from build123d import *

# Parameters (mm, degrees)
SKETCH_1_R      = 2.5
SKETCH_1_R_2    = 2
EXTRUDE_1_DEPTH = 5
SKETCH_2_R      = 2.75
SKETCH_2_R_2    = 2.25
EXTRUDE_2_DEPTH = 6
FILLET_1_R      = 0.1


with BuildPart() as part:
    # Эскиз1 → Вытянуть1 (new body)
    with BuildSketch(Plane.XY):
        Circle(SKETCH_1_R)
        Circle(SKETCH_1_R_2, mode=Mode.SUBTRACT)
    extrude(amount=EXTRUDE_1_DEPTH)

    # Эскиз2 → Вытянуть2 (add)
    with BuildSketch(Plane.XY.offset(5)):
        Circle(SKETCH_2_R)
        Circle(SKETCH_2_R_2, mode=Mode.SUBTRACT)
    extrude(amount=EXTRUDE_2_DEPTH)

    # Скругление1
    fillet_1_edges = [part.edges().sort_by_distance(p)[0] for p in [
        (-2.5, 0, 0),
        (-2.5, 0, 5),
        (-2.75, 0, 5),
    ]]
    fillet(fillet_1_edges, radius=FILLET_1_R)


solid = part.part
Design review of the part built by this model. Coordinates are the model's own, in mm. A direction names the side the tool comes from. Coordinates: 2 decimals unless noted, no trailing zeros. Order: outer loops, then holes, each group sorted by start corner. A loop starts at its lowest first (then second) coordinate and runs counter-clockwise, first axis right, second up.
Item 1: For line 1 (Y direction, x = 0, z = 7.6); line 2 (Y direction, x = 0, z = 1.6); line 3 (X direction, y = -1.5, z = 1.25), list the stretches that pass through material, from the lowest coordinate up.
Item 2: The part is to be moulded in two halves that separate along X. For faces 1 (the cylindrical face through (-0.29, 2.23, 7.96)), 2 (the flat face through (-1, 2, 0)), 3 (the cylindrical face through (-0.596, -2.685, 8.009)), say which applies: pulls with the +X half, pulls with the -X half, needs draft (parallel to the pull), parting line crosses it, or undercut.
Item 3: Take a section at D-D, the plane z = 3.75. Write out the cut boundary in (x, y), then the cut area to 3 significant figures.
Item 4: Take a section at C-C, the plane z = 9.75. Write out the cut boundary in (x, y).
Item 5: For faces 4 (the cylindrical face through (0, -2, 2)), 5 (the cylindrical face through (-0.54, -2.44, 2.47)), list the 3-axis set-ups (+Z, -Z, +X, -X, +Y, -Y) from which the entire face can be reached by the end or side of a thin tool; tool diameter is ignored.
Item 6: Take a section at A-A, the plane y = 0. Write out the cut boundary in (x, z), then the cut area to 3 significant figures.
Item 7: For pin 1 Ø2 at (y, z) = (-0.5, 5) entering from -X; pin 2 Ø2 at (x, z) = (-2, 8.5) entering from -Y; pin 3 Ø2 at (x, y) = (-1, 0.5) entering from +Z; pin 4 Ø1.6 at (x, y) = (0.5, -1) entering from -Z, all flat-tipped, find the tip position at first contact; note any pin that passes through.
The answers:
1. line 1: y = -2.75 to -2.25, 2.25 to 2.75
1. line 2: y = -2.5 to -2, 2 to 2.5
1. line 3: x = -2 to -1.32, 1.32 to 2
2. face 1: undercut
2. face 2: needs draft
2. face 3: parting line crosses it
3. outline: circle Ø5 at (0, 0); hole circle Ø4 at (0, 0)
3. area: 7.07 mm2
4. outline: circle Ø5.5 at (0, 0); hole circle Ø4.5 at (0, 0)
5. face 4: +Z, -Z
5. face 5: -Z
6. outline: (-2.75, 5.1) arc R0.1 ccw to (-2.65, 5) - (-2.6, 5) arc R0.1 cw to (-2.5, 4.9) - (-2.5, 0.1) arc R0.1 ccw to (-2.4, 0) - (-2, 0) - (-2, 5) - (-2.25, 5) - (-2.25, 11) - (-2.75, 11) - close; (2, 0) - (2.4, 0) arc R0.1 ccw to (2.5, 0.1) - (2.5, 4.9) arc R0.1 cw to (2.6, 5) - (2.65, 5) arc R0.1 ccw to (2.75, 5.1) - (2.75, 11) - (2.25, 11) - (2.25, 5) - (2, 5) - close
6. area: 11.0 mm2
7. pin 1: stops at x = -2.75
7. pin 2: stops at y = -2.56
7. pin 3: stops at z = 5
7. pin 4: passes through
